Build history of the part. All positions in model axes, mm. Face numbers are marked on the shaded views. A direction names the side the tool comes from. Give positions to 0.01 mm unless a question says otherwise; leave off trailing zeros. Loops run counter-clockwise (first coordinate to the right, second up) from the corner with the lowest first, then second, coordinate; pieces in that order, holes last. Notation, with made-up numbers: M 78,5.25 L 89,5.25 A15 cw 89,34.25 Z; hole C -4,50 d11. An arc over 180 degrees is marked long. Put each result on its own line as item: value.
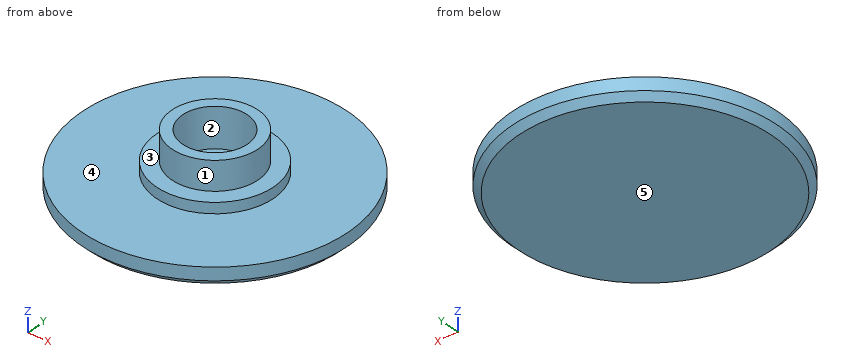
```python
from build123d import *

# Parameters (mm, degrees)
F0_R     = 12.5
F0_R_2   = 5.5
F0_R_3   = 4.05
F1_DEPTH = 1.8
F2_DEPTH = 2.8
F3_DEPTH = 5.5
F4_R     = 3.05
F5_DEPTH = 3.7
F6_SIZE  = 0.6


with BuildPart() as f1:
    # F0 (on Top) → F1 (new body)
    with BuildSketch(Plane.XY):
        Circle(F0_R)
        Circle(F0_R_2, mode=Mode.SUBTRACT)
        Circle(F0_R_2)
        Circle(F0_R_3, mode=Mode.SUBTRACT)
        Circle(F0_R_3)
    extrude(amount=F1_DEPTH)

    # F0 (on Top) → F2 (join)
    with BuildSketch(Plane.XY):
        Circle(F0_R_2)
        Circle(F0_R_3, mode=Mode.SUBTRACT)
    extrude(amount=F2_DEPTH)

    # F0 (on Top) → F3 (join)
    with BuildSketch(Plane.XY):
        Circle(F0_R_3)
    extrude(amount=F3_DEPTH)

    # F4 (on face) → F5 (cut, through all)
    with BuildSketch(Plane.XY.offset(5.5)):
        Circle(F4_R)
    extrude(amount=-F5_DEPTH, mode=Mode.SUBTRACT)

    # F6
    f6_edges = [f1.edges().sort_by_distance(p)[0] for p in [
        (-12.5, 0, 0),
    ]]
    chamfer(f6_edges, length=F6_SIZE)


solid = f1.part
```
Q1. Slice it at B-B (z = 4.15). List the corners of the cut face in (x, y).
Here are the results:
outline: C 0,0 d8.1; hole C 0,0 d6.1
Q2. Tool access for the marked faces 4 and 5: list every direction of +Z, -Z, +X, -X, +Y, -Y with a clear straight run to the whole face (end or side of a thin tool).
Here are the results:
face 4: +Z
face 5: -Z, +X, -X, +Y, -Y
Q3. Drop flat-ended pins along their axis: pin 1 Ø1.8 at (x, y) = (0, 1.5) entering from +Z; pin 2 Ø5.5 at (x, y) = (-0.5, -1) entering from +Z; pin 3 Ø1.5 at (x, z) = (-1, 4) entering from +Y. Give the stop position or say it passes through.
Here are the results:
pin 1: z = 1.8
pin 2: z = 5.5
pin 3: y = 4.04
Q4. Slice it at A-A (y = 0). List the corners of the cut face in (x, z).
Here are the results:
outline: M -12.5,0.6 L -11.9,0 L 11.9,0 L 12.5,0.6 L 12.5,1.8 L 5.5,1.8 L 5.5,2.8 L 4.05,2.8 L 4.05,5.5 L 3.05,5.5 L 3.05,1.8 L -3.05,1.8 L -3.05,5.5 L -4.05,5.5 L -4.05,2.8 L -5.5,2.8 L -5.5,1.8 L -12.5,1.8 Z
Q5. Mould opens along X. For the marked faces 1, 2 and 3 say: pulls with the +X half, pulls with the -X half, needs draft (parallel to the pull), parting line crosses it, or undercut.
Here are the results:
face 1: parting line crosses it
face 2: undercut
face 3: needs draft
Q6. Probe line 1 (Y direction, x = 0, z = 4.05); line 2 (Z direction, x = 3.75, y = -10); line 3 (Y direction, x = -0.25, z = 1.3). List the from-to ranges inside material, lowest first. Write a range as from..to.
Here are the results:
line 1: -4.05..-3.05, 3.05..4.05
line 2: 0..1.8
line 3: -12.5..12.5
